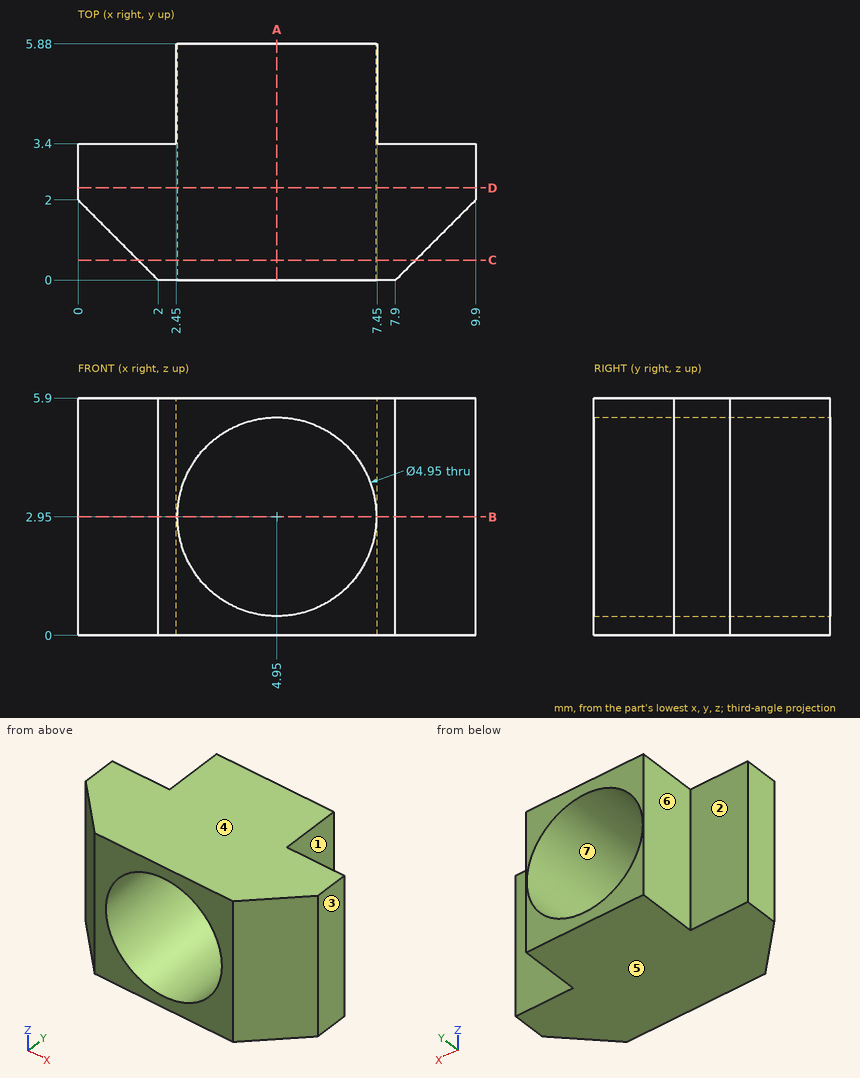
For this review, use the dimensioned drawing (mm, ordinates from the lowest corner) and the shaded views. A direction names the side the tool comes from. Give positions to 0.01 mm unless a question says otherwise; leave off trailing zeros. Write each loop counter-clockwise with the first axis right and the second up, starting at its lowest first coordinate (ties: lowest second). Pieces come first, ordered by that corner, then holes. Notation, with made-up numbers: M 83,77.25 L 112,77.25 A9 cw 112,92.25 Z; hole C -3.75,-29 d6. An arc over 180 degrees is marked long. Answer as a JSON object with one key per item and string values. Group by question number.
Item 1: Consider section C-C on y = 0.5. Write out the cut boundary in (x, z) (3 decimals), plus the area to 3 significant figures.
Item 2: Consider section B-B on z = 2.95. Write out the cut boundary in (x, y) (3 decimals), plus the area to 3 significant figures.
Item 3: Consider section D-D on y = 2.3. Write out the cut boundary in (x, z) (3 decimals).
Item 4: For probe 1 along Z at (x, y) = (4.95, 3.85) (3 decimals); probe 2 along Y at (x, z) = (7.5, 1.9); probe 3 along X at (y, z) = (3, 3.35), list the stretches that pass through material, from the lowest coordinate up. Write a range as [from, to].
Item 5: Tool access review of the marked faces 1, 2 and 3: name each direction out of +Z, -Z, +X, -X, +Y, -Y from which nothing blocks a thin tool from reaching the whole face with its end or side.
Item 6: Draft analysis for pull direction Z (two halves, no side actions). For the marked faces 4, 5, 6 and 7, state which applies: +Z half, -Z half, draft (parallel to the pull), parting line (faces both ways), or undercut.
Item 7: For pin 1 Ø2 at (x, z) = (1, 2) entering from +Y; pin 2 Ø0.7 at (y, z) = (5, 1.5) entering from -X; pin 3 Ø2.5 at (y, z) = (5, 3) entering from +X, all flat-tipped, find the tip position at first contact; note any pin that passes through.
Item 8: Consider section A-A on x = 4.95. Write out the cut boundary in (y, z) (3 decimals), plus the area to 3 significant figures.
Check result:
{
 "1": {"outline": "M 1.5,0 L 8.4,0 L 8.4,5.9 L 1.5,5.9 Z; hole C 4.95,2.95 d4.95", "area": "21.5 mm^2"},
 "2": {"outline": "M 0,2 L 2,0 L 2.475,0 L 2.475,5.88 L 2.45,5.88 L 2.45,3.4 L 0,3.4 Z; M 7.425,0 L 7.9,0 L 9.9,2 L 9.9,3.4 L 7.45,3.4 L 7.45,5.88 L 7.425,5.88 Z", "area": "13.0 mm^2"},
 "3": {"outline": "M 0,0 L 9.9,0 L 9.9,5.9 L 0,5.9 Z; hole C 4.95,2.95 d4.95"},
 "4": {"probe 1": "z = [0, 0.475], [5.425, 5.9]", "probe 2": "y = [0, 3.4]", "probe 3": "x = [0, 2.51], [7.39, 9.9]"},
 "5": {"face 1": "+Z, -Z, +X, +Y", "face 2": "+Z, -Z, -X, +Y", "face 3": "+Z, -Z, +X, +Y, -Y"},
 "6": {"face 4": "+Z half", "face 5": "-Z half", "face 6": "draft", "face 7": "undercut"},
 "7": {"pin 1": "stops at y = 3.4", "pin 2": "stops at x = 2.45", "pin 3": "stops at x = 7.45"},
 "8": {"outline": "M 0,0 L 5.88,0 L 5.88,0.475 L 0,0.475 Z; M 0,5.425 L 5.88,5.425 L 5.88,5.9 L 0,5.9 Z", "area": "5.59 mm^2"}
}
